Autodesk Inventor part; units mm, degrees
ref_plane "YZ Plane" through (0, 0, 0) normal (1, 0, 0) x (0, 1, 0)
ref_plane "XZ Plane" through (0, 0, 0) normal (0, 1, 0) x (-1, 0, 0)
ref_plane "XY Plane" through (0, 0, 0) normal (0, 0, 1) x (1, 0, 0)
sketch "Sketch1" plane through (0, 0, 0) normal (0, 1, 0) x (-1, 0, 0)
  line L0 (-6, 11) -> (-6, -11)
  line L1 (-6, -11) -> (6, -11)
  line L2 (6, -11) -> (6, 11)
  line L3 (6, 11) -> (-6, 11)
  line L4 (-6, 11) -> (6, -11) construction
  line L5 (-6, -11) -> (6, 11) construction
  point P0 (0, 0)
  dimension "d0" = 22
  dimension "d1" = 12
extrude "Extrusion1" add sketch "Sketch1" along normal blind 16
sketch "Sketch2" plane through (0, 16, 0) normal (0, 1, 0) x (1, 0, 0)
  line L0 (6, -16) -> (6, 16)
  line L1 (6, 16) -> (-6, 16)
  line L2 (-6, 16) -> (-6, -16)
  line L3 (-6, -16) -> (6, -16)
  line L4 (6, -16) -> (-6, 16) construction
  line L5 (6, 16) -> (-6, -16) construction
  point P0 (0, 0)
  dimension "d4" = 32
extrude "Extrusion2" add sketch "Sketch2" along normal blind 2
sketch "Sketch3" plane through (0, 18, 0) normal (0, 1, 0) x (1, 0, 0)
  line L0 (6, -11) -> (6, 11)
  line L1 (6, 11) -> (-6, 11)
  line L2 (-6, 11) -> (-6, -11)
  line L3 (-6, -11) -> (6, -11)
  line L4 (6, -11) -> (-6, 11) construction
  line L5 (6, 11) -> (-6, -11) construction
  point P0 (0, 0)
extrude "Extrusion3" add sketch "Sketch3" along normal blind 4
sketch "Sketch4" plane through (0, 22, 0) normal (0, 1, 0) x (1, 0, 0)
  line L0 (6, 11) -> (-6, 11)
  line L1 (0, 11) -> (0, 5)
  circle A0 centre (0, 5) radius 6
  line L2 (-6, -11) -> (6, -11)
  line L3 (0, -11) -> (0, -1)
  circle A1 centre (0, -1) radius 2.5
  point P0 (0, 0)
  dimension "d9" = 6
  dimension "d10" = 10
  dimension "d11" = 5
extrude "Extrusion4" add sketch "Sketch4" along normal blind 4
sketch "Sketch5" plane through (0, 26, 0) normal (0, 1, 0) x (1, 0, 0)
  circle A0 centre (0, 5) radius 2.5
  point P0 (0, 0)
  dimension "d14" = 5
extrude "Extrusion5" add sketch "Sketch5" along normal blind 4
sketch "Sketch6" plane through (0, 30, -5) normal (0, 1, 0) x (1, 0, 0)
  point P0 (0, -5)
  point P1 (0, 0)
hole "Hole1" at (0, 30, -5) direction (0, -1, 0) diameter 1.8 depth 8 tip angle 118
fillet "Fillet1" radius 0.5 1 edges at (-2.5, 30, -5)
fillet "Fillet2" radius 0.5 9 edges at (6, 20, 11) (6, 8, 11) (-6, 8, 11) (-6, 20, 11) (6, 20, -11) (6, 8, -11) (6, 17, 16) (-6, 17, 16) (6, 17, -16)
fillet "Fillet3" radius 0.5 2 edges at (-6, 20, -11) (-6, 8, -11)
fillet "Fillet4" radius 0.5 2 edges at (-2.4451, 24, 0.4792) (2.4451, 24, 0.4792)
sketch "Sketch7" plane through (5.5, 0, -11) normal (0, 0, -1) x (-1, 0, 0)
  line L0 (5.5, 0) -> (5.5, 5)
  circle A0 centre (5.5, 5) radius 0.635
  line L1 (5.5, 5) -> (4.23, 5)
  circle A1 centre (4.23, 5) radius 0.635
  line L2 (5.5, 5) -> (6.77, 5)
  circle A2 centre (6.77, 5) radius 0.635
  dimension "d28" = 5
  dimension "d29" = 1.27
  dimension "d30" = 1.27
  dimension "d31" = 1.27
extrude "Extrusion6" add sketch "Sketch7" along normal blind 10
fillet "Fillet5" radius 0.5 1 edges at (-6, 17, -16)
sketch "Sketch8" plane through (0, 18, 0) normal (0, 1, 0) x (1, 0, 0)
  line L0 (5.5, 16) -> (-5.5, 16)
  line L1 (0, 16) -> (0, 14)
  line L2 (-5.5, -16) -> (5.5, -16)
  line L3 (0, -16) -> (0, -14)
  point P0 (0, 0)
  dimension "d35" = 2
  dimension "d36" = 2
hole "Hole2" at (0, 18, 14) at (0, 18, -14) direction (0, -1, 0) diameter 2.4 depth 3 tip angle 118
properties part number "9g-micro-server"
Design review of the part built by this model. Coordinates are the model's own, in mm. A direction names the side the tool comes from. Give positions to 0.01 mm unless a question says otherwise; leave off trailing zeros. Write each loop counter-clockwise with the first axis right and the second up, starting at its lowest first coordinate (ties: lowest second). Pieces come first, ordered by that corner, then holes. Notation, with made-up numbers: M -24,42.5 L 19,42.5 A24 ccw 19,66.5 Z; hole C 23.25,-3.75 d4. An arc over 180 degrees is marked long. Return JSON: item names as keys, results as strings. Group by question number.
Item 1: Clearance check with flat-ended pins moving along their axes: pin 1 Ø2 at (x, y) = (1, 21) entering from +Z; pin 2 Ø1 at (x, z) = (-1, -9) entering from +Y; pin 3 Ø6 at (x, z) = (-2, 13) entering from -Y; pin 4 Ø2 at (x, y) = (-1, 17.5) entering from -Z. State where each tip first meets the part, or that it passes through.
Item 2: Take a section at D-D (z = 2). Give the boundary of the cut face in (x, y).
Item 3: Take a section at C-C (y = 7.75). Give the boundary of the cut face in (x, z), plus the area to 3 significant figures.
Item 4: Tool access review of faces 5 (the flat face through (0, 26, -2)), 6 (the flat face through (-5, 22, -10)), 7 (the flat face through (0, 20, -11)), 8 (the flat face through (0, 5, -21)): name each direction out of +Z, -Z, +X, -X, +Y, -Y from which nothing blocks a thin tool from reaching the whole face with its end or side.
Item 5: Take a section at B-B (x = 3.5). Give the boundary of the cut face in (y, z), plus the area to 3 significant figures.
Item 6: The part is to be moulded in two halves that separate along X. For faces 1 (the cylindrical face through (1.41, 5.62, -15.93)), 2 (the flat face through (6, 11, -3)), 3 (the cylindrical face through (-0.36, 16.986, -12.855)), 4 (the flat face through (0, 20, 11)), say which applies: pulls with the +X half, pulls with the -X half, needs draft (parallel to the pull), parting line crosses it, or undercut.
Item 7: Wall thickness on line 1 along Z through (x, y) = (0, 16.8); line 2 along X through (y, z) = (24.25, -5); line 3 along X through (y, z) = (16.5, 14): over which ranges is each line inside the solid? List them lowest first.
Return value:
{
 "1": {"pin 1": "stops at z = 11", "pin 2": "stops at y = 26", "pin 3": "stops at y = 0", "pin 4": "stops at z = -16"},
 "2": {"outline": "M -6,0 L 6,0 L 6,22 L 2.29,22 L 2.29,26 L -2.29,26 L -2.29,22 L -6,22 Z"},
 "3": {"outline": "M -6,-10.5 A0.5 ccw -5.5,-11 L 5.5,-11 A0.5 ccw 6,-10.5 L 6,10.5 A0.5 ccw 5.5,11 L -5.5,11 A0.5 ccw -6,10.5 Z", "area": "264 mm2"},
 "4": {"face 5": "+Y", "face 6": "-Z, -X, +Y", "face 7": "-Z, +X, -X, +Y", "face 8": "-Z, +X, -X, +Y, -Y"},
 "5": {"outline": "M 0,-11 L 16,-11 L 16,-16 L 18,-16 L 18,-11 L 22,-11 L 22,-9.87 L 26,-9.87 L 26,-0.13 L 22,-0.13 L 22,11 L 18,11 L 18,16 L 16,16 L 16,11 L 0,11 Z", "area": "543 mm2"},
 "6": {"face 1": "undercut", "face 2": "pulls with the +X half", "face 3": "undercut", "face 4": "needs draft"},
 "7": {"line 1": "z = -16 to -15.2, -12.8 to 12.8, 15.2 to 16", "line 2": "x = -6 to -0.9, 0.9 to 6", "line 3": "x = -6 to -1.2, 1.2 to 6"}
}
